from build123d import *

# Parameters (mm, degrees)
ESQUISSE1_W              = 300
ESQUISSE1_H              = 153
BOSS_EXTRU_1_DEPTH       = 10
ESQUISSE7_R              = 15
ENL_V_MAT_EXTRU_5_DEPTH  = 11
ESQUISSE8_R              = 15
ENL_V_MAT_EXTRU_6_DEPTH  = 11
ESQUISSE9_R              = 15
ENL_V_MAT_EXTRU_7_DEPTH  = 11
ESQUISSE10_R             = 15
ENL_V_MAT_EXTRU_8_DEPTH  = 11
ESQUISSE11_R             = 15
ENL_V_MAT_EXTRU_9_DEPTH  = 11
ESQUISSE12_R             = 15
ENL_V_MAT_EXTRU_10_DEPTH = 11
ESQUISSE13_R             = 15
ENL_V_MAT_EXTRU_11_DEPTH = 11
ESQUISSE14_R             = 15
ENL_V_MAT_EXTRU_12_DEPTH = 11
ESQUISSE16_R             = 12
ENL_V_MAT_EXTRU_14_DEPTH = 11
ESQUISSE17_R             = 12
ENL_V_MAT_EXTRU_15_DEPTH = 11
ESQUISSE2_R              = 4.5
ENL_V_MAT_EXTRU_16_DEPTH = 11


with BuildPart() as part:
    # Esquisse1 → Boss.-Extru.1 (new body)
    with BuildSketch(Plane.XY):
        with Locations((150, 76.5)):
            Rectangle(ESQUISSE1_W, ESQUISSE1_H)
    extrude(amount=BOSS_EXTRU_1_DEPTH)

    # Esquisse7 → Enlèv. mat.-Extru.5 (cut, through all)
    with BuildSketch(Plane.XY.offset(10)):
        with Locations((171, 96.5)):
            Circle(ESQUISSE7_R)
    extrude(amount=-ENL_V_MAT_EXTRU_5_DEPTH, mode=Mode.SUBTRACT)

    # Esquisse8 → Enlèv. mat.-Extru.6 (cut, through all)
    with BuildSketch(Plane.XY.offset(10)):
        with Locations((207, 119)):
            Circle(ESQUISSE8_R)
    extrude(amount=-ENL_V_MAT_EXTRU_6_DEPTH, mode=Mode.SUBTRACT)

    # Esquisse9 → Enlèv. mat.-Extru.7 (cut, through all)
    with BuildSketch(Plane.XY.offset(10)):
        with Locations((243, 119)):
            Circle(ESQUISSE9_R)
    extrude(amount=-ENL_V_MAT_EXTRU_7_DEPTH, mode=Mode.SUBTRACT)

    # Esquisse10 → Enlèv. mat.-Extru.8 (cut, through all)
    with BuildSketch(Plane.XY.offset(10)):
        with Locations((279, 119)):
            Circle(ESQUISSE10_R)
    extrude(amount=-ENL_V_MAT_EXTRU_8_DEPTH, mode=Mode.SUBTRACT)

    # Esquisse11 → Enlèv. mat.-Extru.9 (cut, through all)
    with BuildSketch(Plane.XY.offset(10)):
        with Locations((171, 38.2)):
            Circle(ESQUISSE11_R)
    extrude(amount=-ENL_V_MAT_EXTRU_9_DEPTH, mode=Mode.SUBTRACT)

    # Esquisse12 → Enlèv. mat.-Extru.10 (cut, through all)
    with BuildSketch(Plane.XY.offset(10)):
        with Locations((207, 56.5)):
            Circle(ESQUISSE12_R)
    extrude(amount=-ENL_V_MAT_EXTRU_10_DEPTH, mode=Mode.SUBTRACT)

    # Esquisse13 → Enlèv. mat.-Extru.11 (cut, through all)
    with BuildSketch(Plane.XY.offset(10)):
        with Locations((243, 56.5)):
            Circle(ESQUISSE13_R)
    extrude(amount=-ENL_V_MAT_EXTRU_11_DEPTH, mode=Mode.SUBTRACT)

    # Esquisse14 → Enlèv. mat.-Extru.12 (cut, through all)
    with BuildSketch(Plane.XY.offset(10)):
        with Locations((279, 56.5)):
            Circle(ESQUISSE14_R)
    extrude(amount=-ENL_V_MAT_EXTRU_12_DEPTH, mode=Mode.SUBTRACT)

    # Esquisse16 → Enlèv. mat.-Extru.14 (cut, through all)
    with BuildSketch(Plane.XY.offset(10)):
        with Locations((165, 138)):
            Circle(ESQUISSE16_R)
    extrude(amount=-ENL_V_MAT_EXTRU_14_DEPTH, mode=Mode.SUBTRACT)

    # Esquisse17 → Enlèv. mat.-Extru.15 (cut, through all)
    with BuildSketch(Plane.XY.offset(10)):
        with Locations((135, 138)):
            Circle(ESQUISSE17_R)
    extrude(amount=-ENL_V_MAT_EXTRU_15_DEPTH, mode=Mode.SUBTRACT)

    # Esquisse2 → Enlèv. mat.-Extru.16 (cut, through all)
    with BuildSketch(Plane.XY.offset(10)):
        with Locations((75, 76.5)):
            Circle(ESQUISSE2_R)
    extrude(amount=-ENL_V_MAT_EXTRU_16_DEPTH, mode=Mode.SUBTRACT)


solid = part.part
CAD build for the part. Positions are in the model's coordinates, mm. Coordinates: 2 decimals unless noted, no trailing zeros. Order: outer loops, then holes, each group sorted by start corner. A loop starts at its lowest first (then second) coordinate and runs counter-clockwise, first axis right, second up. Notation, with made-up numbers: (30.25, -32.5) -> (58.25, -32.5) arc R25 cw to (58.25, -12.5) -> close; hole circle Ø10 at (9, -36.75). An arc over 180 degrees is marked (long way). Answer in a Markdown table with one row per item.
1) Band-saw the part on D-D (x = 135). List the corners of the cut face in (y, z), and give its area (3 significant figures).
Check values:
| item | result |
|---|---|
| outline | (0, 0) -> (126, 0) -> (126, 10) -> (0, 10) -> close; (150, 0) -> (153, 0) -> (153, 10) -> (150, 10) -> close |
| area | 1,290 mm2 |
2) Drill centre lines: line 1 (Y direction, x = 207, z = 8.25); line 2 (Y direction, x = 75, z = 3.75); line 3 (X direction, y = 118, z = 4). Where is each one in solid material? Low to high.
Check values:
| item | result |
|---|---|
| line 1 | 0 to 41.5, 71.5 to 104, 134 to 153 |
| line 2 | 0 to 72, 81 to 153 |
| line 3 | 0 to 192.03, 221.97 to 228.03, 257.97 to 264.03, 293.97 to 300 |
3) Band-saw the part on A-A (x = 279). List the corners of the cut face in (y, z), and give its area (3 significant figures).
Check values:
| item | result |
|---|---|
| outline | (0, 0) -> (41.5, 0) -> (41.5, 10) -> (0, 10) -> close; (71.5, 0) -> (104, 0) -> (104, 10) -> (71.5, 10) -> close; (134, 0) -> (153, 0) -> (153, 10) -> (134, 10) -> close |
| area | 930 mm2 |
4) Band-saw the part on C-C (z = 8). Give the number of separate pieces and of enclosed holes in the cut face, and give its area (3 significant figures).
Check values:
| item | result |
|---|---|
| separate pieces | 1 |
| enclosed holes | 11 |
| area | 39,300 mm2 |
5) Band-saw the part on B-B (y = 96.5). List the corners of the cut face in (x, z), and give its area (3 significant figures).
Check values:
| item | result |
|---|---|
| outline | (0, 0) -> (156, 0) -> (156, 10) -> (0, 10) -> close; (186, 0) -> (300, 0) -> (300, 10) -> (186, 10) -> close |
| area | 2,700 mm2 |
